Autodesk Inventor part; units mm, degrees
ref_plane "YZ Plane" through (0, 0, 0) normal (1, 0, 0) x (0, 1, 0)
ref_plane "XZ Plane" through (0, 0, 0) normal (0, 1, 0) x (-1, 0, 0)
ref_plane "XY Plane" through (0, 0, 0) normal (0, 0, 1) x (1, 0, 0)
sketch "Sketch1" plane through (0, 0, 0) normal (0, 1, 0) x (-1, 0, 0)
  line L0 (171.45, 127) -> (-171.45, 127)
  line L1 (-171.45, 127) -> (-171.45, -127)
  line L2 (-171.45, -127) -> (171.45, -127)
  line L3 (171.45, -127) -> (171.45, 127)
  line L4 (171.45, 127) -> (-171.45, -127) construction
  line L5 (-171.45, 127) -> (171.45, -127) construction
  point P0 (0, 0)
  dimension "d0" = 342.9
  dimension "d1" = 254
extrude "Extrusion1" add sketch "Sketch1" along normal blind 25.4
sketch "Sketch6" plane through (171.45, 0, 127) normal (1, 0, 0) x (0, 0, -1)
  line L0 (0, 25.4) -> (254, 25.4)
  line L1 (254, 0) -> (254, 25.4)
  point P0 (127, 0)
  point P1 (228.6, 12.7)
  dimension "d18" = 25.4
  dimension "d19" = 12.7
hole "Hole2" at (171.45, 12.7, -101.6) direction (-1, 0, 0) diameter 12.7 depth 12.7
sketch "Sketch8" plane through (-171.45, 0, -127) normal (-1, 0, 0) x (0, 0, 1)
  circle A0 centre (25.4, 12.7) radius 6.35
  point P0 (127, 0)
hole "Hole3" at (-171.45, 12.7, -101.6) direction (1, 0, 0) diameter 12.7 depth 12.7
properties part number "STEP"
Source: CAD feature listing. Evaluate the final solid. Frame: model axes, mm. A direction names the side the tool comes from. Coordinates: 2 decimals unless noted, no trailing zeros. Loops run counter-clockwise (first coordinate to the right, second up) from the corner with the lowest first, then second, coordinate; pieces in that order, holes last. Notation, with made-up numbers: (36.5, 4.25) - (56.5, 4.25) arc R14 cw to (56.5, 17.25) - close; hole circle Ø11 at (81.5, 59.5). An arc over 180 degrees is marked (long way). One line per item, written item: value. Start each with the question number.
1. Mould query, pull axis Y, two halves, no side actions, for faces 4 (the flat face through (-2, 13, 127)), 5 (the flat face through (2, 25.4, 2)), 6 (the flat face through (158.75, 13, -102)). Classes: pulls with the +Y half, pulls with the -Y half, needs draft (parallel to the pull), parting line crosses it, or undercut.
2. Contact query for flat-ended pins moving along their axis: P1, Ø4, axis at y = 15, z = -103.5, coming from the -X side; P2, Ø4, axis at y = 12.5, z = -101, coming from the +X side. Output: stop coordinate, or through.
3. Section A-A (z = -101.6). Return the cut outline in (x, y).
4. Ray query, L1, parallel to Z at x = -166, y = 12.7; L2, parallel to Y at x = -166.75, z = -101.6. Return the intervals inside material, ascending.
5. Set-up query: faces 1 (the flat face through (2, 0, 2)), 2 (the cylindrical face through (165.011, 15.132, -107.466)), 3 (the cylindrical face through (-165.011, 12.421, -107.944)). Return all of +Z, -Z, +X, -X, +Y, -Y with unobstructed straight access to the full face (end or side cutting, diameter ignored); none if empty.
Verdict:
1. face 4: needs draft
1. face 5: pulls with the +Y half
1. face 6: undercut
2. P1: stops at x = -158.75
2. P2: stops at x = 158.75
3. outline: (-171.45, 0) - (171.45, 0) - (171.45, 6.35) - (158.75, 6.35) - (158.75, 19.05) - (171.45, 19.05) - (171.45, 25.4) - (-171.45, 25.4) - (-171.45, 19.05) - (-158.75, 19.05) - (-158.75, 6.35) - (-171.45, 6.35) - close
4. L1: z = -127 to -107.95, -95.25 to 127
4. L2: y = 0 to 6.35, 19.05 to 25.4
5. face 1: +Z, -Z, +X, -X, -Y
5. face 2: +X
5. face 3: -X
